Study the drawing (mm; zero at the part's minimum x, y, z) and answer. A direction names the side the tool comes from. Round coordinates to 2 decimals unless told otherwise and drop trailing zeros. Order: outer loops, then holes, each group sorted by start corner. A loop starts at its lowest first (then second) coordinate and runs counter-clockwise, first axis right, second up. Notation, with made-up numbers: (42.5, 68) -> (91.5, 68) arc R26 ccw to (91.5, 82) -> close; hole circle Ø3 at (-29, 17). An arc over 180 degrees is marked (long way). Answer in a Markdown table with one row per item. Add a question column.
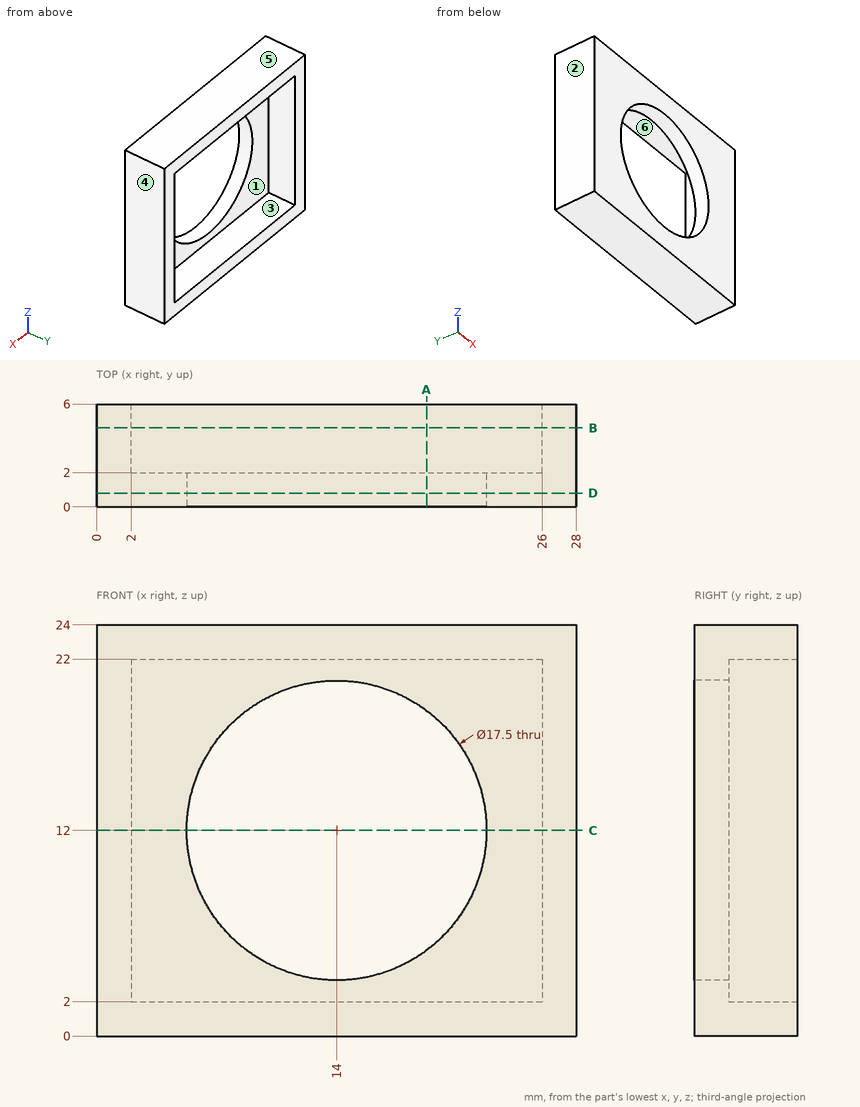
Item 1: Find the intervals of material crossed by probe 1 along Z at (x, y) = (24.75, 2.85); probe 2 along X at (y, z) = (3.6, 12.5); probe 3 along Z at (x, y) = (14, 0.95), in increasing order. Write a range as [from, to].
Item 2: The part is cut by section A-A, the plane x = 19.25. Give the vertices of the cut face in (y, z).
Item 3: A tool of negligible diameter and unlimited length cuts with its end or side. For the marked faces 1 and 2, from which of +Z, -Z, +X, -X, +Y, -Y can it reach the whole face along a straight path? Write none if from no direction.
Item 4: The part is cut by section B-B, the plane y = 4.6. Give the vertices of the cut face in (x, z), and give its area (3 significant figures).
Item 5: The part is cut by section D-D, the plane y = 0.8. Give the vertices of the cut face in (x, z), and give its area (3 significant figures).
Item 6: For a pull along X with two mould halves and no side action, classify the marked faces 3, 4, 5 and 6 as released by +X, released by -X, zero draft, split by the parting line, or undercut.
Item 7: The part is cut by section C-C, the plane z = 12. Give the vertices of the cut face in (x, y), and give its area (3 significant figures).
Resolved:
| question | item | result |
|---|---|---|
| 1 | probe 1 | [0, 2], [22, 24] |
| 1 | probe 2 | [0, 2], [26, 28] |
| 1 | probe 3 | [0, 3.25], [20.75, 24] |
| 2 | outline | (0, 0) -> (6, 0) -> (6, 2) -> (2, 2) -> (2, 5) -> (0, 5) -> close; (0, 19) -> (2, 19) -> (2, 22) -> (6, 22) -> (6, 24) -> (0, 24) -> close |
| 3 | face 1 | +Y |
| 3 | face 2 | +Z, -Z, -X, +Y, -Y |
| 4 | outline | (0, 0) -> (28, 0) -> (28, 24) -> (0, 24) -> close; hole (2, 2) -> (26, 2) -> (26, 22) -> (2, 22) -> close |
| 4 | area | 192 mm2 |
| 5 | outline | (0, 0) -> (28, 0) -> (28, 24) -> (0, 24) -> close; hole circle Ø17.5 at (14, 12) |
| 5 | area | 431 mm2 |
| 6 | face 3 | undercut |
| 6 | face 4 | released by +X |
| 6 | face 5 | zero draft |
| 6 | face 6 | undercut |
| 7 | outline | (0, 0) -> (5.25, 0) -> (5.25, 2) -> (2, 2) -> (2, 6) -> (0, 6) -> close; (22.75, 0) -> (28, 0) -> (28, 6) -> (26, 6) -> (26, 2) -> (22.75, 2) -> close |
| 7 | area | 37.0 mm2 |
